Verification items for the finished model (mm, model axes). A direction names the side the tool comes from. Round coordinates to 2 decimals unless told otherwise and drop trailing zeros. Loops run counter-clockwise (first coordinate to the right, second up) from the corner with the lowest first, then second, coordinate; pieces in that order, holes last. Notation, with made-up numbers: M -6,8.5 L 1,8.5 A25 ccw 1,35.5 Z; hole C 81.25,4.25 d1. An arc over 180 degrees is marked long. One line per item, written item: value.
from build123d import *

# Parameters (mm, degrees)
SKETCH1_R           = 3
BOSS_EXTRUDE1_DEPTH = 27.5
SKETCH3_R           = 18
CUT_EXTRUDE1_DEPTH  = 1
SKETCH4_R           = 5
CUT_EXTRUDE2_DEPTH  = 28.5
SKETCH5_R           = 15
SKETCH5_R_2         = 5
BOSS_EXTRUDE2_DEPTH = 16
FILLET1_R           = 1
CUT_EXTRUDE3_REACH  = 47
SKETCH6_R           = 3


with BuildPart() as part:
    # Sketch1 → Boss-Extrude1 (new body)
    with BuildSketch(Plane.XY):
        with BuildLine():
            Line((0, 40), (0, 5))
            ThreePointArc((0, 5), (-1.464466094, 1.464466094), (-5, 0))
            Line((-5, 0), (-40, 0))
            ThreePointArc((-40, 0), (-43.535533906, 1.464466094), (-45, 5))
            Line((-45, 5), (-45, 40))
            ThreePointArc((-45, 40), (-43.535533906, 43.535533906), (-40, 45))
            Line((-40, 45), (-5, 45))
            ThreePointArc((-5, 45), (-1.464466094, 43.535533906), (0, 40))
        make_face()
        with Locations((-6, 39)):
            Circle(SKETCH1_R, mode=Mode.SUBTRACT)
        with Locations((-6, 6)):
            Circle(SKETCH1_R, mode=Mode.SUBTRACT)
        with Locations((-39, 6)):
            Circle(SKETCH1_R, mode=Mode.SUBTRACT)
        with Locations((-39, 39)):
            Circle(SKETCH1_R, mode=Mode.SUBTRACT)
    extrude(amount=BOSS_EXTRUDE1_DEPTH)

    # Sketch3 → Cut-Extrude1 (cut)
    with BuildSketch(Plane.XY.offset(27.5)):
        with Locations((-22.5, 22.5)):
            Circle(SKETCH3_R)
    extrude(amount=-CUT_EXTRUDE1_DEPTH, mode=Mode.SUBTRACT)

    # Sketch4 → Cut-Extrude2 (cut, through all)
    with BuildSketch(Plane(origin=(0, 0, 0), x_dir=(-1, 0, 0), z_dir=(0, 0, -1))):
        with Locations((22.5, 22.5)):
            Circle(SKETCH4_R)
    extrude(amount=-CUT_EXTRUDE2_DEPTH, mode=Mode.SUBTRACT)

    # Sketch5 → Boss-Extrude2 (add)
    with BuildSketch(Plane(origin=(0, 0, 0), x_dir=(-1, 0, 0), z_dir=(0, 0, -1))):
        with Locations((22.5, 22.5)):
            Circle(SKETCH5_R)
        with Locations((22.5, 22.5)):
            Circle(SKETCH5_R_2, mode=Mode.SUBTRACT)
    extrude(amount=BOSS_EXTRUDE2_DEPTH)

    # Fillet1
    fillet1_edges = [part.edges().sort_by_distance(p)[0] for p in [
        (-7.5, 22.5, -16),
    ]]
    fillet(fillet1_edges, radius=FILLET1_R)

    # Sketch6 → Cut-Extrude3 (cut, up to next)
    with BuildSketch(Plane(origin=(0, 45, 0), x_dir=(1, 0, 0), z_dir=(0, 1, 0)), mode=Mode.PRIVATE) as cut_extrude3_sk1:
        with Locations((-22.5, -14)):
            Circle(SKETCH6_R)
    cut_extrude3_tool1 = extrude(cut_extrude3_sk1.sketch, amount=-CUT_EXTRUDE3_REACH, mode=Mode.PRIVATE) & part.part
    add(cut_extrude3_tool1.solids().sort_by_distance((-22.5, 45, 14))[0], mode=Mode.SUBTRACT)


solid = part.part
(1) Depth check by flat-ended pin: pin 1 Ø3.5 at (x, y) = (-6, 6) entering from -Z; pin 2 Ø1.5 at (x, y) = (-36.5, 27.5) entering from -Z; pin 3 Ø8 at (x, y) = (-39, 39) entering from -Z; pin 4 Ø1.5 at (x, y) = (-30, 7) entering from +Z. Enter the tip coordinate at first touch or a pass-through.
Completed:
pin 1: passes through
pin 2: stops at z = -15.99
pin 3: stops at z = 0
pin 4: stops at z = 26.5
(2) Thickness scan on L1, parallel to Y at x = -22.5, z = 18.25; L2, parallel to X at y = 33.5, z = 14; L3, parallel to X at y = 8, z = 4. Record the ranges inside material, lowest first. Write a range as from..to.
Completed:
L1: y = 0..17.5, 27.5..45
L2: x = -45..-25.5, -19.5..0
L3: x = -45..-41.24, -36.76..-8.24, -3.76..0
(3) Sectioned sample at B-B on x = -22.5. Enter the section's corners in (y, z), and give its area (3 significant figures).
Completed:
outline: M 0,0 L 7.5,0 L 7.5,-15 A1 ccw 8.5,-16 L 17.5,-16 L 17.5,26.5 L 4.5,26.5 L 4.5,27.5 L 0,27.5 Z; M 27.5,-16 L 36.5,-16 A1 ccw 37.5,-15 L 37.5,0 L 45,0 L 45,11 L 27.5,11 Z; M 27.5,17 L 45,17 L 45,27.5 L 40.5,27.5 L 40.5,26.5 L 27.5,26.5 Z
area: 1,150 mm^2
(4) Sectioned sample at D-D on y = 39. Enter the section's corners in (x, z).
Completed:
outline: M -45,0 L -42,0 L -42,27.5 L -45,27.5 Z; M -36,0 L -9,0 L -9,27.5 L -15.31,27.5 L -15.31,26.5 L -29.69,26.5 L -29.69,27.5 L -36,27.5 Z; M -3,0 L 0,0 L 0,27.5 L -3,27.5 Z; hole C -22.5,14 d6
(5) Mould release check, pull along Y, two halves, no side actions. Record for faces 6 (the face through (-2, 44, 14)), 7 (the face through (-19.248, 7.857, -7.395)), 8 (the face through (-26.402, 4.928, 27.007)), 9 (the face through (0, 23, 14)): +Y half, -Y half, draft (parallel to the pull), parting line (faces both ways), or undercut.
Completed:
face 6: +Y half
face 7: parting line
face 8: undercut
face 9: draft
(6) Sectioned sample at A-A on y = 22.5. Enter the section's corners in (x, z).
Completed:
outline: M -45,0 L -37.5,0 L -37.5,-15 A1 ccw -36.5,-16 L -27.5,-16 L -27.5,26.5 L -40.5,26.5 L -40.5,27.5 L -45,27.5 Z; M -17.5,-16 L -8.5,-16 A1 ccw -7.5,-15 L -7.5,0 L 0,0 L 0,27.5 L -4.5,27.5 L -4.5,26.5 L -17.5,26.5 Z
(7) Tool access check on faces 1 (the face through (-4.616, 3.338, 13.558)), 2 (the face through (-43, 1, 14)), 3 (the face through (-22, 38, 0)), 4 (the face through (-18.8, 18.8, 26.5)), 5 (the face through (-24.9, 35.9, 15.8)). Record the directions out of +Z, -Z, +X, -X, +Y, -Y that give a thin tool (end or side, any length) a straight path to the whole face; none if there is none.
Completed:
face 1: +Z, -Z
face 2: +Z, -Z, -X, -Y
face 3: -Z
face 4: +Z
face 5: +Y
(8) Sectioned sample at C-C on z = 3. Enter the section's corners in (x, y), and give its area (3 significant figures).
Completed:
outline: M -45,5 A5 ccw -40,0 L -5,0 A5 ccw 0,5 L 0,40 A5 ccw -5,45 L -40,45 A5 ccw -45,40 Z; hole C -39,6 d6; hole C -39,39 d6; hole C -22.5,22.5 d10; hole C -6,6 d6; hole C -6,39 d6
area: 1,810 mm^2
